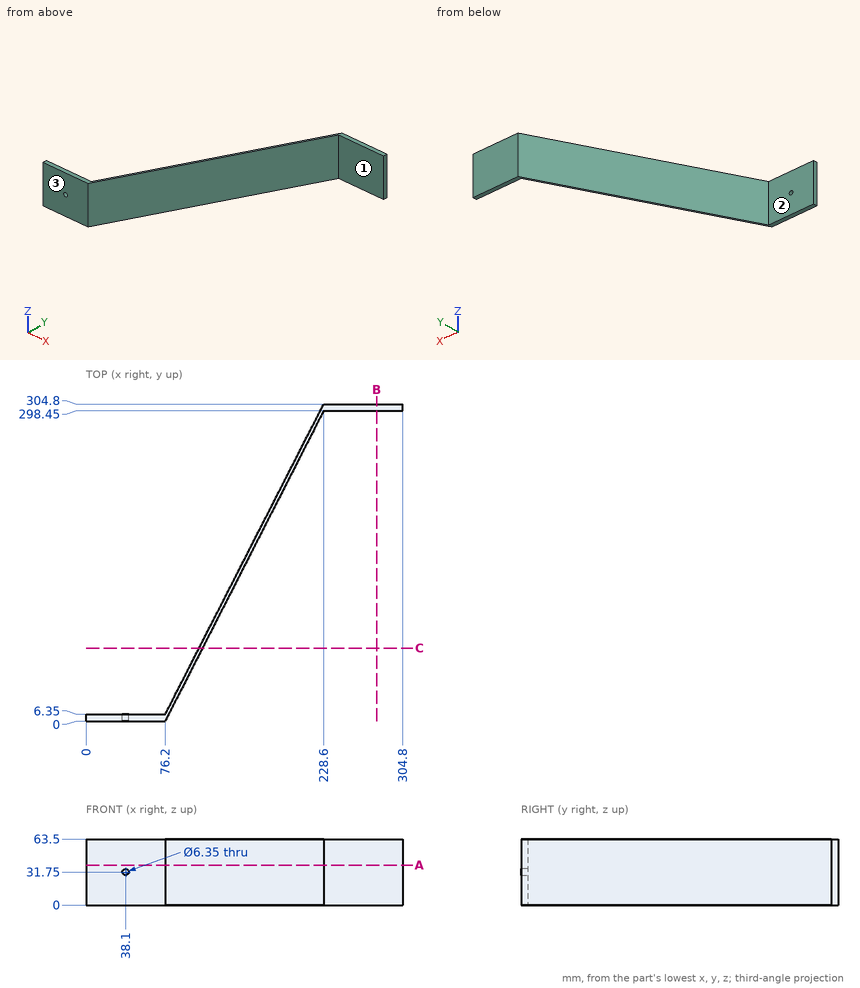
Here's the drawing with two shaded views (mm, measured from the low corner). I have some questions. A direction names the side the tool comes from. Give positions to 0.01 mm unless a question says otherwise; leave off trailing zeros. Loops run counter-clockwise (first coordinate to the right, second up) from the corner with the lowest first, then second, coordinate; pieces in that order, holes last. Notation, with made-up numbers: (6, 28) - (54, 28) arc R28 cw to (54, 60) - close; hole circle Ø5 at (34, 26.25). An arc over 180 degrees is marked (long way). One line per item, written item: value.
(1) If we section it at B-B, the plane x = 279.5: List the corners of the cut face in (y, z) for me, plus the area to 3 significant figures.
Verdict:
outline: (298.45, 0) - (304.8, 0) - (304.8, 63.5) - (298.45, 63.5) - close
area: 403 mm^2
(2) If we section it at A-A, the plane z = 38.5: List the corners of the cut face in (x, y) for me.
Verdict:
outline: (0, 0) - (76.2, 0) - (228.6, 298.45) - (304.8, 298.45) - (304.8, 304.8) - (228.6, 304.8) - (76.2, 6.35) - (0, 6.35) - close
(3) I'm going to push flat-ended pins straight in: pin 1 (2 mm diameter, centred on y = 126.5, z = 42, fed in from -X); pin 2 (5 mm diameter, centred on x = 38.1, z = 31.75, fed in from -Y); pin 3 (6 mm diameter, centred on y = 272, z = 17.5, fed in from -X); pin 4 (1 mm diameter, centred on y = 178, z = 37.5, fed in from -X). Where does each tip first touch, or does it pass through?
Verdict:
pin 1: x = 137.04
pin 2: through
pin 3: x = 210.32
pin 4: x = 163.6
(4) If we section it at C-C, the plane y = 70: List the corners of the cut face in (x, z) for me, plus the area to 3 significant figures.
Verdict:
outline: (108.7, 0) - (111.94, 0) - (111.94, 63.5) - (108.7, 63.5) - close
area: 206 mm^2
(5) I need wall thicknesses on line 1 along Z through (x, y) = (38, 3); line 2 along X through (y, z) = (5, 31); line 3 along Y through (x, z) = (36, 29). Which ranges of each line are inside material? Lowest first, please.
Verdict:
line 1: 0 to 28.58, 34.92 to 63.5
line 2: 0 to 35.01, 41.19 to 78.75
line 3: 0 to 6.35
(6) On a 3-axis mill with a long thin cutter (end or side, diameter ignored), from which of +Z, -Z, +X, -X, +Y, -Y can I reach the whole of each face in a straight line? I mean the marked faces 1, 2 and 3. Say none if no direction works.
Verdict:
face 1: +Z, -Z, +X, -Y
face 2: +Z, -Z, -X, +Y
face 3: +Z, -Z, +X, -X, -Y
